Here's how the part is built. I have some questions about the finished solid (model axes, mm). A direction names the side the tool comes from. Coordinates: 2 decimals unless noted, no trailing zeros. Write each loop counter-clockwise with the first axis right and the second up, starting at its lowest first coordinate (ties: lowest second). Pieces come first, ordered by that corner, then holes. Notation, with made-up numbers: (38.25, -2) -> (57.25, -2) arc R14 ccw to (57.25, 5) -> close; hole circle Ø1 at (38.25, 67.25). An arc over 180 degrees is marked (long way). Use a Markdown table: item, result. Add a question column.
Item 1: Imagine slicing it at C-C, the plane y = 2.2. Write out the boundary of the cut face in (x, z), and give its area (3 significant figures).
Item 2: If we mould it in two halves opening along X, with no side actions, what happens to faces 1 (the cylindrical face through (9.677, -0.479, 6.972)), 2 (the flat face through (2, 2.5, 2)), 3 (the cylindrical face through (-10.19, -2.2, 2.54))? For each: pulls with the +X half, pulls with the -X half, needs draft (parallel to the pull), parting line crosses it, or undercut.
Item 3: On a 3-axis mill with a long thin cutter (end or side, diameter ignored), from which of +Z, -Z, +X, -X, +Y, -Y can I reach the whole of each face in a straight line? I mean faces 4 (the flat face through (14.522, 0, 2)), 5 (the cylindrical face through (3.274, 0.055, 6.972)). Say none if no direction works.
Item 4: Will this pin go through, and if not, where does the flat tip stop? pin 1 Ø2 at (x, y) = (-1.5, 1) entering from +Z.
Item 5: If I drill on line 1 along Z through (x, y) = (-1, -0.9); line 2 along X through (y, z) = (-0.65, 8); line 3 along X through (y, z) = (-0.8, 9), over which ranges is the centre line in solid material (lowest first)? Write a range as from..to.
Item 6: Imagine slicing it at B-B, the plane x = 2. Write out the boundary of the cut face in (y, z).
Item 7: Imagine slicing it at A-A, the plane z = 7.5. Write out the boundary of the cut face in (x, y), and give its area (3 significant figures).
```python
from build123d import *

# Parameters (mm, degrees)
F0_W     = 25
F0_H     = 5
F1_DEPTH = 5
F2_R     = 1.25
F3_DEPTH = 5
F4_R     = 1


with BuildPart() as f1:
    # F0 (on Top) → F1 (new body)
    with BuildSketch(Plane.XY):
        with Locations((2.022313, 0)):
            Rectangle(F0_W, F0_H)
    extrude(amount=F1_DEPTH)

    # F2 (on face) → F3 (join)
    with BuildSketch(Plane.XY.offset(5)):
        with Locations((4.522313, 0)):
            Circle(F2_R)
        with Locations((8.522313, 0)):
            Circle(F2_R)
    extrude(amount=F3_DEPTH)

    # F4
    f4_edges = [f1.edges().sort_by_distance(p)[0] for p in [
        (-10.477687, -2.5, 2.5),
        (-10.477687, 2.5, 2.5),
        (3.272313, 0, 10),
        (7.272313, 0, 10),
        (-10.477687, 0, 0),
    ]]
    fillet(f4_edges, radius=F4_R)


solid = f1.part
```
Ans:
| question | item | result |
|---|---|---|
| 1 | outline | (-10.19, 0.3) arc R1 ccw to (-9.48, 0) -> (14.52, 0) -> (14.52, 5) -> (-10.19, 5) -> close |
| 1 | area | 124 mm^2 |
| 2 | face 1 | undercut |
| 2 | face 2 | needs draft |
| 2 | face 3 | pulls with the -X half |
| 3 | face 4 | +Z, -Z, +X, +Y, -Y |
| 3 | face 5 | +Z |
| 4 | pin 1 | stops at z = 5 |
| 5 | line 1 | z = 0..5 |
| 5 | line 2 | x = 3.45..5.59, 7.45..9.59 |
| 5 | line 3 | x = 3.56..5.48, 7.56..9.48 |
| 6 | outline | (-2.5, 0) -> (2.5, 0) -> (2.5, 5) -> (-2.5, 5) -> close |
| 7 | outline | circle Ø2.5 at (4.52, 0); circle Ø2.5 at (8.52, 0) |
| 7 | area | 9.82 mm^2 |
